Verification items for the finished model (mm, model axes). A direction names the side the tool comes from. Coordinates: 2 decimals unless noted, no trailing zeros. Write each loop counter-clockwise with the first axis right and the second up, starting at its lowest first coordinate (ties: lowest second). Pieces come first, ordered by that corner, then holes. Notation, with made-up numbers: (26, 17) -> (43, 17) arc R9 ccw to (43, 32) -> close; hole circle Ø10 at (31, 38). An arc over 180 degrees is marked (long way). Use CSV: the item, a comma, the result in double quotes.
```python
from build123d import *
from OCP.BRepFilletAPI import BRepFilletAPI_MakeChamfer

# Parameters (mm, degrees)
SKETCH_1_W          = 41
SKETCH_1_H          = 60
SKETCH_1_R          = 2.3
SKETCH_1_R_2        = 1.9
EXTRUDE_1_DEPTH     = 3
CHAMFER_1_SIZE      = 2
SKETCH_2_W          = 41
SKETCH_2_H          = 60
SKETCH_2_W_2        = 38
SKETCH_2_H_2        = 57
EXTRUDE_1_2_DEPTH   = 18
SKETCH_3_W          = 27
SKETCH_3_H          = 3.030341357
CUT_EXTRUDE_1_DEPTH = 18
SKETCH_4_R          = 2.5
EXTRUDE_2_DEPTH     = 18
SKETCH_5_R          = 1.55
CUT_EXTRUDE_2_DEPTH = 10
SKETCH_7_W          = 7
SKETCH_7_H          = 4.356080651
CUT_EXTRUDE_3_DEPTH = 1.2
FILLET_2_R          = 0.5
FILLET_3_R          = 2
CHAMFER_4_SIZE      = 0.866025404
CHAMFER_4_SIZE_2    = 1.5
CHAMFER_6_SIZE      = 0.5
CHAMFER_6_SIZE2     = 0.288675135
SKETCH_8_W          = 4
SKETCH_8_H          = 5
EXTRUDE_3_DEPTH     = 10
FILLET_6_R          = 1
FILLET_7_R          = 2
FILLET_8_R          = 0.5
CHAMFER_7_SIZE      = 1


with BuildPart() as part:
    # Эскиз1 → Extrude 1 (new body)
    with BuildSketch(Plane(origin=(0, 0, 0), x_dir=(1, 0, 0), z_dir=(0, 1, 0))):
        Rectangle(SKETCH_1_W, SKETCH_1_H)
        with Locations(Location((0, 24, 0), (0, 0, 270))):
            Circle(SKETCH_1_R, mode=Mode.SUBTRACT)
        with Locations(Location((0, -24, 0), (0, 0, 270))):
            Circle(SKETCH_1_R, mode=Mode.SUBTRACT)
        with Locations(Location((0, -12, 0), (0, 0, 270))):
            Circle(SKETCH_1_R_2, mode=Mode.SUBTRACT)
    extrude(amount=EXTRUDE_1_DEPTH)

    # Фаска1
    chamfer_1_edges = [part.edges().sort_by_distance(p)[0] for p in [
        (0, 3, -26.3),
        (0, 3, 21.7),
    ]]
    chamfer(chamfer_1_edges, length=CHAMFER_1_SIZE)

    # Эскиз2 → Extrude 1 2 (add)
    with BuildSketch(Plane(origin=(0, 3, 0), x_dir=(1, 0, 0), z_dir=(0, 1, 0))):
        Rectangle(SKETCH_2_W, SKETCH_2_H)
        Rectangle(SKETCH_2_W_2, SKETCH_2_H_2, mode=Mode.SUBTRACT)
    extrude(amount=EXTRUDE_1_2_DEPTH)

    # Эскиз3 → Вырез-Вытянуть1 (cut)
    with BuildSketch(Plane(origin=(0, 21, 0), x_dir=(1, 0, 0), z_dir=(0, 1, 0))):
        with Locations((0, 29.478101209)):
            Rectangle(SKETCH_3_W, SKETCH_3_H)
    extrude(amount=-CUT_EXTRUDE_1_DEPTH, mode=Mode.SUBTRACT)

    # Эскиз4 → Бобышка-Вытянуть2 (add)
    with BuildSketch(Plane(origin=(0, 3, 0), x_dir=(1, 0, 0), z_dir=(0, 1, 0))):
        with Locations((17, 25)):
            Circle(SKETCH_4_R)
        with Locations((-17, 25)):
            Circle(SKETCH_4_R)
        with Locations((17, -25)):
            Circle(SKETCH_4_R)
        with Locations((-17, -25)):
            Circle(SKETCH_4_R)
    extrude(amount=EXTRUDE_2_DEPTH)

    # Эскиз5 → Вырез-Вытянуть2 (cut)
    with BuildSketch(Plane(origin=(0, 21, 0), x_dir=(1, 0, 0), z_dir=(0, 1, 0))):
        with Locations(Location((17, 25, 0), (0, 0, 270))):
            Circle(SKETCH_5_R)
        with Locations(Location((17, -25, 0), (0, 0, 270))):
            Circle(SKETCH_5_R)
        with Locations(Location((-17, -25, 0), (0, 0, 270))):
            Circle(SKETCH_5_R)
        with Locations(Location((-17, 25, 0), (0, 0, 270))):
            Circle(SKETCH_5_R)
    extrude(amount=-CUT_EXTRUDE_2_DEPTH, mode=Mode.SUBTRACT)

    # Эскиз7 → Вырез-Вытянуть3 (cut)
    with BuildSketch(Plane(origin=(0, 21, 0), x_dir=(1, 0, 0), z_dir=(0, 1, 0))):
        with Locations((0, -28.804800006)):
            Rectangle(SKETCH_7_W, SKETCH_7_H)
    extrude(amount=-CUT_EXTRUDE_3_DEPTH, mode=Mode.SUBTRACT)

    # Скругление2
    fillet_2_edges = [part.edges().sort_by_distance(p)[0] for p in [
        (-3.5, 20.4, 28.5),
        (3.5, 20.4, 28.5),
        (3.5, 20.4, 30),
        (-3.5, 20.4, 30),
    ]]
    fillet(fillet_2_edges, radius=FILLET_2_R)

    # Скругление3
    fillet_3_edges = [part.edges().sort_by_distance(p)[0] for p in [
        (20.5, 10.5, 30),
        (-20.5, 10.5, 30),
        (-20.5, 10.5, -30),
        (20.5, 10.5, -30),
    ]]
    fillet(fillet_3_edges, radius=FILLET_3_R)

    # Фаска4
    # the kernel refuses this chamfer: 1.5, 0.866025404 mm, written as the material it takes off along each edge
    with BuildSketch(Plane(origin=(0, 0, 24), x_dir=(0, 0, 1), z_dir=(-1, 0, 0))) as chamfer_4_piece_1:
        Polygon((2.3 + CHAMFER_4_SIZE, 0), (2.3, CHAMFER_4_SIZE_2), (2.3, 0), align=None)
    revolve(axis=Axis((0, 0, 24), (0, 1, 0)), mode=Mode.SUBTRACT)
    with BuildSketch(Plane(origin=(18.5, 0, -30), x_dir=(0, -0.01932676561270073, 0.999813220622208), z_dir=(-1, 0, 0))) as chamfer_4_piece_2:
        Polygon((CHAMFER_4_SIZE_2 * 0.999813220622, CHAMFER_4_SIZE_2 * 0.0193267656127), (-CHAMFER_4_SIZE * 0.0193267656079, CHAMFER_4_SIZE * 0.999813220373), (0, 0), align=None)
    extrude(amount=37, mode=Mode.SUBTRACT)
    with BuildSketch(Plane(origin=(-20.5, 0, -28), x_dir=(0.999813220622208, -0.01932676561270073, 0), z_dir=(0, 0, 1)), Plane(origin=(20.5, 0, 28), x_dir=(-0.999813220622208, -0.01932676561270073, 0), z_dir=(0, 0, -1))) as chamfer_4_piece_3:
        Polygon((CHAMFER_4_SIZE_2 * 0.999813220622, CHAMFER_4_SIZE_2 * 0.0193267656127), (-CHAMFER_4_SIZE * 0.0193267656079, CHAMFER_4_SIZE * 0.999813220373), (0, 0), align=None)
    extrude(amount=56, mode=Mode.SUBTRACT)
    with BuildSketch(Plane(origin=(-18.5, 0, 30), x_dir=(0, 0.9983227437537924, 0.0578938624026721), z_dir=(1, 0, 0))) as chamfer_4_piece_4:
        Polygon((CHAMFER_4_SIZE * 0.998322743505, -CHAMFER_4_SIZE * 0.0578938623883), (-CHAMFER_4_SIZE_2 * 0.0578938624027, -CHAMFER_4_SIZE_2 * 0.998322743754), (0, 0), align=None)
    extrude(amount=37, mode=Mode.SUBTRACT)
    with BuildSketch(Plane(origin=(-18.5, 0, -28), x_dir=(0, 0, -1), z_dir=(1, 0, 0))) as chamfer_4_piece_5:
        Polygon((2 - CHAMFER_4_SIZE_2, 0), (2, CHAMFER_4_SIZE), (2, 0), align=None)
    revolve(axis=Axis((-18.5, 0, -28), (0, 1, 0)), revolution_arc=90, mode=Mode.SUBTRACT)
    with BuildSketch(Plane(origin=(-18.5, 0, 28), x_dir=(0, 0, 1), z_dir=(1, 0, 0))) as chamfer_4_piece_6:
        Polygon((2 - CHAMFER_4_SIZE_2, 0), (2, -CHAMFER_4_SIZE), (2, 0), align=None)
    revolve(axis=Axis((-18.5, 0, 28), (0, -1, 0)), revolution_arc=90, mode=Mode.SUBTRACT)
    with BuildSketch(Plane(origin=(18.5, 0, 28), x_dir=(0, 0, 1), z_dir=(-1, 0, 0))) as chamfer_4_piece_7:
        Polygon((2, CHAMFER_4_SIZE), (2 - CHAMFER_4_SIZE_2, 0), (2, 0), align=None)
    revolve(axis=Axis((18.5, 0, 28), (0, 1, 0)), revolution_arc=90, mode=Mode.SUBTRACT)
    with BuildSketch(Plane(origin=(18.5, 0, -28), x_dir=(0, 0, -1), z_dir=(-1, 0, 0))) as chamfer_4_piece_8:
        Polygon((2 - CHAMFER_4_SIZE_2, 0), (2, -CHAMFER_4_SIZE), (2, 0), align=None)
    revolve(axis=Axis((18.5, 0, -28), (0, -1, 0)), revolution_arc=90, mode=Mode.SUBTRACT)
    with BuildSketch(Plane(origin=(0, 0, -24), x_dir=(0, 0, 1), z_dir=(-1, 0, 0))) as chamfer_4_piece_9:
        Polygon((2.3 + CHAMFER_4_SIZE, 0), (2.3, CHAMFER_4_SIZE_2), (2.3, 0), align=None)
    revolve(axis=Axis((0, 0, -24), (0, 1, 0)), mode=Mode.SUBTRACT)
    with BuildSketch(Plane(origin=(0, 0, 12), x_dir=(0, 0, 1), z_dir=(-1, 0, 0))) as chamfer_4_piece_10:
        Polygon((1.9 + CHAMFER_4_SIZE, 0), (1.9, CHAMFER_4_SIZE_2), (1.9, 0), align=None)
    revolve(axis=Axis((0, 0, 12), (0, 1, 0)), mode=Mode.SUBTRACT)

    # Фаска6: one chamfer whose edges measure the first distance from different faces: ONE call of the kernel's chamfer builder (chamfer() names one face for all edges)
    chamfer_6_edges_1 = [part.edges().sort_by_distance(p)[0] for p in [
        (-17, 21, -26.55),
        (-17, 21, 23.45),
    ]]
    chamfer_6_side_1 = [part.faces().sort_by_distance(p)[0] for p in [
        (-11.25, 21, 29.376381527),
    ]]
    chamfer_6_edges_2 = [part.edges().sort_by_distance(p)[0] for p in [
        (17, 21, 23.45),
        (17, 21, -26.55),
    ]]
    chamfer_6_side_2 = [part.faces().sort_by_distance(p)[0] for p in [
        (11.25, 21, 29.376381527),
    ]]
    chamfer_6 = BRepFilletAPI_MakeChamfer(part.part.solid().wrapped)
    for e in chamfer_6_edges_1:
        chamfer_6.Add(CHAMFER_6_SIZE, CHAMFER_6_SIZE2, e.wrapped, chamfer_6_side_1[0].wrapped)  # the first distance lies on this face
    for e in chamfer_6_edges_2:
        chamfer_6.Add(CHAMFER_6_SIZE, CHAMFER_6_SIZE2, e.wrapped, chamfer_6_side_2[0].wrapped)  # the first distance lies on this face
    add(Compound.cast(chamfer_6.Shape()), mode=Mode.REPLACE)

    # Эскиз8 → Бобышка-Вытянуть3 (add)
    with BuildSketch(Plane(origin=(0, 3, 0), x_dir=(1, 0, 0), z_dir=(0, 1, 0))):
        with Locations((17, -14)):
            Rectangle(SKETCH_8_W, SKETCH_8_H)
        with Locations((-17, -5.5)):
            Rectangle(SKETCH_8_W, SKETCH_8_H)
    extrude(amount=EXTRUDE_3_DEPTH)

    # Скругление6
    fillet_6_edges = [part.edges().sort_by_distance(p)[0] for p in [
        (19, 8, 16.5),
        (17, 3, 11.5),
        (19, 8, 11.5),
        (15, 3, 14),
        (15, 8, 11.5),
        (17, 3, 16.5),
        (15, 8, 16.5),
        (19, 13, 14),
        (17, 13, 11.5),
        (15, 13, 14),
        (17, 13, 16.5),
        (-19, 8, 3),
        (-17, 3, 8),
        (-19, 8, 8),
        (-15, 3, 5.5),
        (-15, 8, 8),
        (-17, 3, 3),
        (-15, 8, 3),
        (-19, 13, 5.5),
        (-17, 13, 8),
        (-15, 13, 5.5),
        (-17, 13, 3),
    ]]
    fillet(fillet_6_edges, radius=FILLET_6_R)

    # Скругление7
    fillet_7_edges = [part.edges().sort_by_distance(p)[0] for p in [
        (-13.5, 3, -29.25),
        (13.5, 3, -29.25),
    ]]
    fillet(fillet_7_edges, radius=FILLET_7_R)

    # Скругление8
    fillet_8_edges = [part.edges().sort_by_distance(p)[0] for p in [
        (0, 3, -30),
        (13.5, 13, -30),
        (12.914213562, 3.585786438, -30),
        (-12.914213562, 3.585786438, -30),
        (-13.5, 13, -30),
    ]]
    fillet(fillet_8_edges, radius=FILLET_8_R)

    # Фаска7
    chamfer_7_edges = [part.edges().sort_by_distance(p)[0] for p in [
        (0, 3, 10.1),
    ]]
    chamfer(chamfer_7_edges, length=CHAMFER_7_SIZE)


solid = part.part
```
1) Set-up check for faces 1 (the cylindrical face through (-15.463, 15.924, -25.202)), 2 (the flat face through (20.5, 11, 0)), 3 (the cylindrical face through (12.9, 3.57, -29.01)): record each of +Z, -Z, +X, -X, +Y, -Y from which the full face is reachable in a straight line by a thin tool's end or side.
Return value:
face 1,"+Y"
face 2,"+Z, -Z, +X, +Y, -Y"
face 3,"-Z, +Y"
2) Gauge pin test, flat ends, axial feed: pin 1 (1 mm diameter, centred on x = -13, z = -22.5, fed in from +Y); pin 2 (1.9 mm diameter, centred on x = -17, z = 25, fed in from +Y); pin 3 (0.6 mm diameter, centred on x = 17, z = 14.5, fed in from +Y). Record the tip position at first contact, or that the pin passes through.
Return value:
pin 1,"y = 3"
pin 2,"y = 11"
pin 3,"y = 13"
3) Cross-section at A-A (z = -4.5). Record the boundary of the cut face in (x, y), plus the area to 3 significant figures.
Return value:
outline,"(-20.5, 0.87) -> (-19, 0) -> (19, 0) -> (20.5, 0.87) -> (20.5, 21) -> (19, 21) -> (19, 3) -> (-19, 3) -> (-19, 21) -> (-20.5, 21) -> close"
area,"176 mm2"
4) Cross-section at C-C (z = 5.5). Record the boundary of the cut face in (x, y), plus the area to 3 significant figures.
Return value:
outline,"(-20.5, 0.87) -> (-19, 0) -> (19, 0) -> (20.5, 0.87) -> (20.5, 21) -> (19, 21) -> (19, 3) -> (-14, 3) arc R1 cw to (-15, 4) -> (-15, 12) arc R1 ccw to (-16, 13) -> (-18, 13) arc R1 cw to (-19, 14) -> (-19, 21) -> (-20.5, 21) -> close"
area,"216 mm2"
5) Mould release check, pull along X, two halves, no side actions. Record for faces 4 (the cylindrical face through (-19.93, 11.07, 29.4)), 5 (the flat face through (-16, 12, -28.5)), 6 (the conical face through (19.25, 0.33, 28.77)): released by +X, released by -X, zero draft, split by the parting line, or undercut.
Return value:
face 4,"released by -X"
face 5,"undercut"
face 6,"released by +X"
6) Cross-section at B-B (y = 15). Give the number of separate pieces and of enclosed holes in the cut face, plus the area to 3 significant figures.
Return value:
separate pieces,"1"
enclosed holes,"4"
area,"294 mm2"
7) Scan lines: L1, parallel to X at y = 16.25, z = 25; L2, parallel to X at y = 15.75, z = 10; L3, parallel to X at y = 1.9, z = 12. Record each from-to range of solid material in increasing order.
Return value:
L1,"-20.5 to -18.55, -15.45 to -14.5, 14.5 to 15.45, 18.55 to 20.5"
L2,"-20.5 to -19, 19 to 20.5"
L3,"-20.5 to -1.9, 1.9 to 20.5"
